Autodesk Inventor part; units mm, degrees
ref_plane "YZ Plane" through (0, 0, 0) normal (1, 0, 0) x (0, 1, 0)
ref_plane "XZ Plane" through (0, 0, 0) normal (0, 1, 0) x (-1, 0, 0)
ref_plane "XY Plane" through (0, 0, 0) normal (0, 0, 1) x (1, 0, 0)
sketch "Sketch1" plane through (0, 0, 0) normal (0, 1, 0) x (-1, 0, 0)
  circle A0 centre (18.5, 28) radius 23.85
  circle A1 centre (37, -23.25) radius 13.85
  circle A2 centre (-35, -38.75) radius 13.85
  circle A3 centre (-30.9, 25.8) radius 13.85
  circle A4 centre (0, -23.25) radius 13.85
  line L0 (56.25, 58.25) -> (-56.25, 58.25)
  line L1 (-56.25, -58.25) -> (56.25, -58.25)
  line L2 (0, -105.9299) -> (0, 123.2086) construction
  line L3 (-76.4777, -38.75) -> (-5.35, -38.75) construction
  line L4 (-123.5447, -23.25) -> (82.5572, -23.25) construction
  line L5 (56.25, -58.25) -> (56.25, 58.25)
  line L6 (56.25, 58.25) -> (56.25, -58.25)
  line L7 (-56.25, 58.25) -> (-56.25, -58.25)
  line L8 (100.0459, 28) -> (-13.85, 28) construction
  line L9 (-9.7154, 25.8) -> (-68.4996, 25.8) construction
  line L10 (18.5, 82.6038) -> (18.5, -4.654) construction
  line L11 (-30.9, 82.6038) -> (-30.9, 8.6393) construction
  point P0 (0, 0)
  point P1 (0, 0)
  dimension "d0" = 47.7
  dimension "d1" = 27.7
  dimension "d2" = 27.7
  dimension "d3" = 27.7
  dimension "d4" = 27.7
  dimension "d7" = 37
  dimension "d9" = 30.9
  dimension "d10" = 19.5
  dimension "d11" = 35
  dimension "d12" = 35
  dimension "d13" = 25.8
  dimension "d14" = 28
  dimension "d15" = 56.25
  dimension "d16" = 58.25
  dimension "d17" = 116.5
  dimension "d18" = 112.5
  dimension "d19" = 18.5
  dimension "d20" = 32.45
extrude "Extrusion1" add sketch "Sketch1" along normal blind 5
sketch "Sketch2" plane through (0, 5, 0) normal (0, 1, 0) x (1, 0, 0)
  line L0 (-56.25, 58.25) -> (-56.25, -58.25)
  line L1 (-56.25, -58.25) -> (56.25, -58.25)
  line L2 (56.25, -58.25) -> (56.25, 58.25)
  line L3 (56.25, 58.25) -> (-56.25, 58.25)
  circle A0 centre (0, 23.25) radius 13.85
  circle A1 centre (30.9, -25.8) radius 13.85
  circle A2 centre (35, 38.75) radius 13.85
  circle A3 centre (-37, 23.25) radius 13.85
  circle A4 centre (-18.5, -28) radius 23.85
  line L4 (-56.25, 58.25) -> (-56.25, -58.25)
  line L5 (-56.25, 23.25) -> (15.75, 23.25)
  line L6 (19.75, 38.75) -> (56.25, 38.75)
  line L7 (56.25, -58.25) -> (56.25, 58.25)
  line L8 (17.75, 25.25) -> (17.75, 36.75)
  arc A5 (15.75, 23.25) -> (17.75, 25.25) centre (15.75, 25.25) ccw
  arc A6 (19.75, 38.75) -> (17.75, 36.75) centre (19.75, 36.75) ccw
  point P0 (0, 0)
  point P1 (17.75, 23.25)
  point P2 (17.75, 38.75)
  point P3 (-50.85, 23.25)
  point P4 (-23.15, 23.25)
  point P5 (-13.85, 23.25)
  point P6 (13.85, 23.25)
  point P7 (21.15, 38.75)
  point P8 (48.85, 38.75)
  dimension "d23" = 74
  dimension "d25" = 38.5
  dimension "d26" = 2
  dimension "d27" = 35
  dimension "d28" = 19.5
sketch "Sketch3" plane through (0, 5, 0) normal (0, 1, 0) x (1, 0, 0)
  line L0 (-56.25, -28) -> (8.75, -28)
  line L1 (12.3221, -25.8) -> (56.25, -25.8)
  line L2 (-56.25, 58.25) -> (-56.25, -58.25)
  line L3 (-56.25, -58.25) -> (56.25, -58.25)
  line L4 (56.25, -58.25) -> (56.25, 58.25)
  line L5 (56.25, 58.25) -> (-56.25, 58.25)
  circle A0 centre (0, 23.25) radius 13.85
  circle A1 centre (30.9, -25.8) radius 13.85
  circle A2 centre (35, 38.75) radius 13.85
  circle A3 centre (-37, 23.25) radius 13.85
  circle A4 centre (-18.5, -28) radius 23.85
  line L6 (56.25, -58.25) -> (56.25, 58.25)
  line L7 (-56.25, 58.25) -> (-56.25, -58.25)
  line L8 (10.75, -26) -> (10.75, -25.8)
  arc A5 (8.75, -28) -> (10.5361, -26.9) centre (8.75, -26) ccw
  arc A6 (12.3221, -25.8) -> (10.5361, -26.9) centre (12.3221, -27.8) ccw
  point P0 (0, 0)
  point P1 (10.75, -28)
  point P2 (44.75, -25.8)
  point P3 (17.05, -25.8)
  point P4 (5.35, -28)
  point P5 (-42.35, -28)
  dimension "d29" = 67
  dimension "d30" = 2
extrude "Extrusion2" cut sketch "Sketch3" against normal blind 10 contours L0 A5 A6 L1 A1 L4 L3 L2 A4
extrude "Extrusion3" cut sketch "Sketch2" against normal through all contours L3 L2 L6 A2 A6 L8 A5 L5 A0 A3 L0
fillet "Fillet1" radius 4 4 edges at (-56.25, 2.5, -23.25) (-56.25, 2.5, 28) (56.25, 2.5, 25.8) (56.25, 2.5, -38.75)
properties part number "Top Bottle Middle"
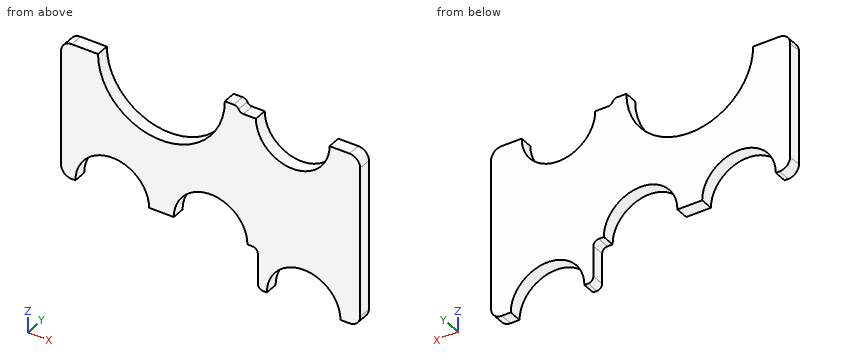
Can you work these out from the model? Positions are in its coordinate system, mm. Give positions to 0.01 mm unless a question says otherwise; leave off trailing zeros. Order: outer loops, then holes, each group sorted by start corner. A loop starts at its lowest first (then second) coordinate and runs counter-clockwise, first axis right, second up. Notation, with made-up numbers: M 67,58.5 L 89,58.5 A29 ccw 89,94.5 Z; hole C 39.5,29 d10. An arc over 180 degrees is marked long. Use one line per item in the form item = value.
Item 1: If we section it at D-D, the plane x = -18.5: Write out the boundary of the cut face in (y, z).
Values follow:
outline = M 0,-23.25 L 5,-23.25 L 5,4.15 L 0,4.15 Z
Item 2: If we section it at C-C, the plane z = 8.5: Write out the boundary of the cut face in (x, y), and give its area (3 significant figures).
Values follow:
outline = M -56.25,0 L -32.23,0 L -32.23,5 L -56.25,5 Z; M -4.77,0 L 56.25,0 L 56.25,5 L -4.77,5 Z
area = 425 mm^2
Item 3: Will these pins go through, and if not, where does the flat tip stop? pin 1 Ø2.5 at (x, y) = (14, 2) entering from +Z; pin 2 Ø2 at (x, y) = (40.5, 1) entering from +Z; pin 3 Ø2.5 at (y, z) = (1.5, -31.5) entering from -X; pin 4 Ø4 at (x, z) = (13.5, 2) entering from -Y.
Values follow:
pin_1 = 25.8
pin_2 = 16.89
pin_3 = 17.75
pin_4 = 0
Item 4: If we section it at B-B, the plane y = 0.8: Write out the boundary of the cut face in (x, z), and give its area (3 significant figures).
Values follow:
outline = M -56.25,-19.25 A4 ccw -52.25,-23.25 L -50.85,-23.25 A13.85 cw -23.15,-23.25 L -13.85,-23.25 A13.85 cw 13.85,-23.25 L 15.75,-23.25 A2 cw 17.75,-25.25 L 17.75,-36.75 A2 ccw 19.75,-38.75 L 21.15,-38.75 A13.85 cw 48.85,-38.75 L 52.25,-38.75 A4 ccw 56.25,-34.75 L 56.25,21.8 A4 ccw 52.25,25.8 L 44.75,25.8 A13.85 cw 17.05,25.8 L 12.32,25.8 A2 cw 10.54,26.9 A2 ccw 8.75,28 L 5.35,28 A23.85 cw -42.35,28 L -52.25,28 A4 ccw -56.25,24 Z
area = 4,150 mm^2
Item 5: If I drill on line 1 along X through (y, z) = (3.4, 18.5); line 2 along X through (y, z) = (1.4, -17); line 3 along X through (y, z) = (2.85, -30.5), over which ranges is the centre line in solid material (lowest first)? Write a range as [from, to].
Values follow:
line_1 = [-56.25, -40.38], [3.38, 19.13], [42.67, 56.25]
line_2 = [-56.25, -49.36], [-24.64, -12.36], [12.36, 56.25]
line_3 = [17.75, 23.88], [46.12, 56.25]
Item 6: If we section it at A-A, the plane z = 20: Write out the boundary of the cut face in (x, y), and give its area (3 significant figures).
Values follow:
outline = M -56.25,0 L -40.97,0 L -40.97,5 L -56.25,5 Z; M 3.97,0 L 18.32,0 L 18.32,5 L 3.97,5 Z; M 43.48,0 L 56.25,0 L 56.25,5 L 43.48,5 Z
area = 212 mm^2
